Autodesk Inventor part; units mm, degrees
ref_plane "YZ Plane" through (0, 0, 0) normal (1, 0, 0) x (0, 1, 0)
ref_plane "XZ Plane" through (0, 0, 0) normal (0, 1, 0) x (-1, 0, 0)
ref_plane "XY Plane" through (0, 0, 0) normal (0, 0, 1) x (1, 0, 0)
sketch "Sketch1" plane through (0, 0, 0) normal (1, 0, 0) x (0, 1, 0)
  line L0 (9.25, 0.0185) -> (11.25, 0.0185)
  line L1 (11.25, 0.0185) -> (11.25, -9.9815)
  line L2 (11.25, -9.9815) -> (11.25, -12)
  arc A0 (1.9984, -22.0011) -> (7.875, -14) centre (-8.063, -8.4526) ccw
  arc A1 (7.9841, -34.947) -> (1.9984, -22.0011) centre (-30.628, -44.9433) ccw
  arc A2 (4, -22) -> (11.25, -12) centre (-13.1002, -1.9743) ccw
  arc A3 (9.9841, -34.947) -> (4, -22) centre (-38.5, -49.5) ccw
  line L3 (7.875, -9.9815) -> (7.875, -14)
  line L4 (0, 0) -> (0, -36)
  line L5 (7.9841, -34.947) -> (0, -34.947)
  line L6 (0, -34.947) -> (0, -35.947)
  line L7 (9.9841, -34.947) -> (9.9841, -35.947)
  line L8 (9.9841, -35.947) -> (0, -35.947)
  line L9 (7.875, -9.9815) -> (0, -9.9815)
  line L10 (0, -9.9815) -> (0, -8.9815)
  line L11 (0, -8.9815) -> (9.25, -8.9815)
  line L12 (9.25, -8.9815) -> (9.25, 0.0185)
  dimension "d26" = 9.25
  dimension "d28" = 2
  dimension "d37" = 34.9656
  dimension "d57" = 36
  dimension "d59" = 1
  dimension "d60" = 1
  dimension "d61" = 90
revolve "Revolution1" add sketch "Sketch1" angle 360 about axis through (0, 0, 0) along (0, 0, -1) contours L0 L1 L2 A2 A3 L7 L8 L4 L5 A1 A0 L3 L9 L11 L12
move or copy body "Move Body1" bodies to move or copy 1 copy no rotation origin (0, 0, 0) rotation axis (1, 0, 0) rotation angle 90
fillet "Fillet6" radius 2 1 edges at (0, 22.0011, -1.9984)
fillet "Fillet7" radius 5 1 edges at (0, 14, -7.875)
fillet "Fillet8" radius 5 1 edges at (0, 12, -11.25)
fillet "Fillet9" radius 5 1 edges at (0, 22, -4)
properties part number "nozzle-cfd" material "ABS Plastic"
Model file for the job. Use its own axes, mm. A direction names the side the tool comes from. Coordinates: 2 decimals unless noted, no trailing zeros. Loops run counter-clockwise (first coordinate to the right, second up) from the corner with the lowest first, then second, coordinate; pieces in that order, holes last. Notation, with made-up numbers: (66.5, -32) - (81.5, -32) arc R33 ccw to (81.5, -4) - close; hole circle Ø2 at (73, -18). An arc over 180 degrees is marked (long way). Answer as a JSON object with one key per item and string values. Group by question number.
(1) Probe line 1 along X through (y, z) = (6, 0); line 2 along Z through (x, y) = (0, 10.9) (3 decimals); line 3 along Y through (x, z) = (-2.25, 0.5). List the from-to ranges inside material, lowest first.
(2) Cut at A-A (z = -6). State how many separate pieces and enclosed holes the cut face has, then the cut area to 3 significant figures.
(3) Flat gauge pins, fed straight in: pin 1 (2 mm diameter, centred on y = 24, z = -0.5, fed in from +X); pin 2 (6 mm diameter, centred on x = -4.5, y = 4.5, fed in from -Z); pin 3 (5 mm diameter, centred on y = 11.5, z = -3.5, fed in from -X). Where does each tip first touch, or does it go through?
(4) Cut at B-B (y = 3). Give the cut face in (x, z).
(5) Tool access for faces 1 (the face through (0, 35.947, 0)), 2 (the face through (7.808, 11.551, -1.025)), 3 (the face through (-6.08, 35.45, -7.92)), 4 (the face through (9.03, 4.42, -2.01)): list every direction of +Z, -Z, +X, -X, +Y, -Y with a clear straight run to the whole face (end or side of a thin tool).
(6) Cut at D-D (y = 9.5). Give the cut face in (x, z).
(7) Two-plate mould, pull along Z, no slides. Class faces 5 (the face through (0, 8.982, 0)), 6 (the face through (-9, -0.018, -3)), 7 (the face through (-9.98, 5.55, 5.19)): released by +Z, released by -Z, zero draft, split by the parting line, or undercut.
Geometry says:
{
 "1": {"line 1": "x = -11.25 to -9.25, 9.25 to 11.25", "line 2": "z = -11.25 to -7.875, 7.875 to 11.25", "line 3": "y = 8.98 to 9.98, 34.95 to 35.95"},
 "2": {"separate pieces": "2", "enclosed holes": "2", "area": "217 mm^2"},
 "3": {"pin 1": "stops at x = 5.79", "pin 2": "stops at z = -11.15", "pin 3": "stops at x = -11.2"},
 "4": {"outline": "circle Ø22.5 at (0, 0); hole circle Ø18.5 at (0, 0)"},
 "5": {"face 1": "+Z, -Z, +X, -X, +Y", "face 2": "none", "face 3": "+Y", "face 4": "-Y"},
 "6": {"outline": "circle Ø22.5 at (0, 0)"},
 "7": {"face 5": "undercut", "face 6": "zero draft", "face 7": "split by the parting line"}
}
